```python
from build123d import *

# Parameters (mm, degrees)
REDONDEO1_R = 1


with BuildPart() as part:
    # Croquis1 → Revolución1 (revolve)
    with BuildSketch(Plane(origin=(0, 0, 0), x_dir=(0, 0, -1), z_dir=(1, 0, 0))):
        Polygon((0, 1.8), (0, 6), (-4.9, 6), (-4.9, 3.5), (-1.6, 3.5), (-1.6, 1.8), align=None)
    revolve(axis=Axis((0, 0, 0), (0, 0, 1)))

    # Redondeo1
    redondeo1_edges = [part.edges().sort_by_distance(p)[0] for p in [
        (0, -6, 4.9),
    ]]
    fillet(redondeo1_edges, radius=REDONDEO1_R)


solid = part.part
```
Geometry check sheet. Reference: the model listing, model coordinates, mm. A direction names the side the tool comes from. Coordinates: 2 decimals unless noted, no trailing zeros. Write each loop counter-clockwise with the first axis right and the second up, starting at its lowest first coordinate (ties: lowest second). Pieces come first, ordered by that corner, then holes. Notation, with made-up numbers: M -12,77 L 2,77 A34 cw 2,107 Z; hole C -10.5,89.5 d4. An arc over 180 degrees is marked long. Answer as a JSON object with one key per item and string values.
1. Draft check along X on faces 3 (the cylindrical face through (1.341, 3.233, 3.227)), 4 (the cylindrical face through (0, -6, 2)), 5 (the flat face through (-1.4, 1.4, 0)). Enter one of: released by +X, released by -X, zero draft, split by the parting line, or undercut.
Answers below:
{"face 3": "undercut", "face 4": "split by the parting line", "face 5": "zero draft"}
2. Tool access check on faces 1 (the cylindrical face through (-0.541, 1.717, 0.789)), 2 (the flat face through (-1, -2, 1.6)). Record the directions out of +Z, -Z, +X, -X, +Y, -Y that give a thin tool (end or side, any length) a straight path to the whole face; none if there is none.
Answers below:
{"face 1": "+Z, -Z", "face 2": "+Z"}
3. Section check A-A, the plane y = 0. Enter the section's corners in (x, z), plus the area to 3 significant figures.
Answers below:
{"outline": "M -6,0 L -1.8,0 L -1.8,1.6 L -3.5,1.6 L -3.5,4.9 L -5,4.9 A1 ccw -6,3.9 Z; M 1.8,0 L 6,0 L 6,3.9 A1 ccw 5,4.9 L 3.5,4.9 L 3.5,1.6 L 1.8,1.6 Z", "area": "29.5 mm²"}
4. Go/stop test with flat-tipped pins: pin 1 Ø1.5 at (y, z) = (-1.5, 3.5) entering from +X; pin 2 Ø1 at (x, z) = (-1, 1.5) entering from +Y; pin 3 Ø2 at (x, z) = (2, 2.5) entering from -Y. Record where each tip stops, or that it passes through.
Answers below:
{"pin 1": "stops at x = 5.95", "pin 2": "stops at y = 5.98", "pin 3": "stops at y = -5.92"}
5. Section check C-C, the plane z = 1.45. Enter the section's corners in (x, y).
Answers below:
{"outline": "C 0,0 d12; hole C 0,0 d3.6"}
6. Section check D-D, the plane z = 2.55. Enter the section's corners in (x, y), plus the area to 3 significant figures.
Answers below:
{"outline": "C 0,0 d12; hole C 0,0 d7", "area": "74.6 mm²"}
7. Scan lines: L1, parallel to Y at x = 0, z = 3.95; L2, parallel to X at y = 0, z = 0.4. Record each from-to range of solid material in increasing order.
Answers below:
{"L1": "y = -6 to -3.5, 3.5 to 6", "L2": "x = -6 to -1.8, 1.8 to 6"}
